from build123d import *

# Parameters (mm, degrees)
EXTRUDE_1_DEPTH     = 8
CUT_EXTRUDE_1_DEPTH = 8
CHAMFER_1_SIZE      = 3


with BuildPart() as part:
    # 스케치1 → 보스-돌출1 (new body)
    with BuildSketch(Plane(origin=(0, 0, 0), x_dir=(1, 0, 0), z_dir=(0, 1, 0))):
        Polygon((0, 0), (0, 20), (35, 20), (35, 0), (30, 0), (30, 8), (5, 8), (5, 0), align=None)
    extrude(amount=EXTRUDE_1_DEPTH)

    # 스케치2 → 컷-돌출1 (cut)
    with BuildSketch(Plane(origin=(0, 8, 0), x_dir=(1, 0, 0), z_dir=(0, 1, 0))):
        with BuildLine():
            Line((29.5, 11.9), (25.5, 11.9))
            ThreePointArc((25.5, 11.9), (23.4, 14), (25.5, 16.1))
            Line((25.5, 16.1), (29.5, 16.1))
            ThreePointArc((29.5, 16.1), (31.6, 14), (29.5, 11.9))
        make_face()
        with BuildLine():
            Line((5.5, 16.1), (9.5, 16.1))
            ThreePointArc((9.5, 16.1), (11.6, 14), (9.5, 11.9))
            Line((9.5, 11.9), (5.5, 11.9))
            ThreePointArc((5.5, 11.9), (3.4, 14), (5.5, 16.1))
        make_face()
    extrude(amount=-CUT_EXTRUDE_1_DEPTH, mode=Mode.SUBTRACT)

    # 모따기1
    chamfer_1_edges = [part.edges().sort_by_distance(p)[0] for p in [
        (0, 4, -20),
        (35, 4, -20),
    ]]
    chamfer(chamfer_1_edges, length=CHAMFER_1_SIZE)


solid = part.part
Work out the finished part from the listing and answer in its coordinate system (mm). A direction names the side the tool comes from. Coordinates: 2 decimals unless noted, no trailing zeros. Write each loop counter-clockwise with the first axis right and the second up, starting at its lowest first coordinate (ties: lowest second). Pieces come first, ordered by that corner, then holes. Notation, with made-up numbers: M 46,9.25 L 62,9.25 A16 ccw 62,27.25 Z; hole C 11,1.5 d6. An arc over 180 degrees is marked long. Write item = value, one per line.
1. For faces 1 (the face through (7, 4, -16.1)), 2 (the face through (3, 4, 0)), 3 (the face through (18, 4, -8)), determine the directions among +Z, -Z, +X, -X, +Y, -Y from which every point of the face is accessible in a straight line to the end or side of a thin tool.
Solution:
face_1 = +Y, -Y
face_2 = +Z, +X, -X, +Y, -Y
face_3 = +Z, +Y, -Y
2. The part is cut by section B-B (z = -3.5). Determine the outline of the cut face in (x, y).
Solution:
outline = M 0,0 L 5,0 L 5,8 L 0,8 Z; M 30,0 L 35,0 L 35,8 L 30,8 Z
3. Straight lines are drawn through the part: line 1 (X direction, y = 5.5, z = -2); line 2 (X direction, y = 2.5, z = -14); line 3 (Z direction, x = 26.5, y = 2.25). For each, find the intervals that lie inside material, in ascending order. Write a range as from..to.
Solution:
line_1 = 0..5, 30..35
line_2 = 0..3.4, 11.6..23.4, 31.6..35
line_3 = -20..-16.1, -11.9..-8
4. The part is cut by section C-C (y = 1). Determine the outline of the cut face in (x, z), then the cut area to 3 significant figures.
Solution:
outline = M 0,-17 L 3,-20 L 32,-20 L 35,-17 L 35,0 L 30,0 L 30,-8 L 5,-8 L 5,0 L 0,0 Z; hole M 5.5,-16.1 L 9.5,-16.1 A2.1 ccw 9.5,-11.9 L 5.5,-11.9 A2.1 ccw Z; hole M 25.5,-16.1 L 29.5,-16.1 A2.1 ccw 29.5,-11.9 L 25.5,-11.9 A2.1 ccw Z
area = 430 mm2
5. The part is cut by section D-D (x = 25). Determine the outline of the cut face in (y, z), then the cut area to 3 significant figures.
Solution:
outline = M 0,-20 L 8,-20 L 8,-16.04 L 0,-16.04 Z; M 0,-11.96 L 8,-11.96 L 8,-8 L 0,-8 Z
area = 63.4 mm2
6. Determine the mould class of faces 4 (the face through (3.4, 4.1, -14)), 5 (the face through (34, 4, -18)), 6 (the face through (35, 4, -9)), 7 (the face through (33, 4, 0)) for opening direction Z: released by +Z, released by -Z, zero draft, split by the parting line, or undercut.
Solution:
face_4 = undercut
face_5 = released by -Z
face_6 = zero draft
face_7 = released by +Z
7. Flat-ended cylindrical pins translate along their axes: pin 1 (4 mm diameter, centred on x = 23.5, y = 6, fed in from +Z); pin 2 (1 mm diameter, centred on x = 29, z = -15, fed in from +Y). Find the tip coordinate at first contact, or state that the pin passes through.
Solution:
pin_1 = -8
pin_2 = through
8. The part is cut by section A-A (z = -14). Determine the outline of the cut face in (x, y), then the cut area to 3 significant figures.
Solution:
outline = M 0,0 L 3.4,0 L 3.4,8 L 0,8 Z; M 11.6,0 L 23.4,0 L 23.4,8 L 11.6,8 Z; M 31.6,0 L 35,0 L 35,8 L 31.6,8 Z
area = 149 mm2
